Verification items for the finished model (mm, model axes). Face numbers are marked on the shaded views. A direction names the side the tool comes from. Give positions to 0.01 mm unless a question says otherwise; leave off trailing zeros. Order: outer loops, then holes, each group sorted by start corner. A loop starts at its lowest first (then second) coordinate and runs counter-clockwise, first axis right, second up. Notation, with made-up numbers: (40, 32.5) -> (74, 32.5) arc R28 cw to (74, 61.5) -> close; hole circle Ø2 at (51.5, 20). An arc over 180 degrees is marked (long way). Return JSON: item names as keys, results as strings. Group by question number.
(1) Depth check by flat-ended pin: pin 1 Ø0.8 at (y, z) = (15.5, 0) entering from +X; pin 2 Ø3 at (x, y) = (-15.5, 1) entering from -Z; pin 3 Ø1.8 at (x, y) = (5.5, 6) entering from -Z; pin 4 Ø1.4 at (x, z) = (-15.5, -0.5) entering from +Y. Enter the tip coordinate at first touch or a pass-through.
(2) Thickness scan on line 1 along Y through (x, z) = (0, -0.9); line 2 along Y through (x, z) = (0, 0.7); line 3 along X through (y, z) = (-1.25, -0.45). Record the ranges inside material, lowest first.
(3) Cross-section at B-B on x = -15.8. Enter the section's corners in (y, z).
(4) Cross-section at A-A on x = 0. Enter the section's corners in (y, z).
(5) Cross-section at D-D on z = 0.55. Enter the section's corners in (x, y), then the cut area to 3 significant figures.
(6) Release check for a two-part mould opening along X. For the marked faces 5, 6 and 7 record: pulls with the +X half, pulls with the -X half, needs draft (parallel to the pull), parting line crosses it, or undercut.
(7) Tool access check on the marked faces 1, 2, 3 and 4. Record the directions out of +Z, -Z, +X, -X, +Y, -Y that give a thin tool (end or side, any length) a straight path to the whole face; none if there is none.
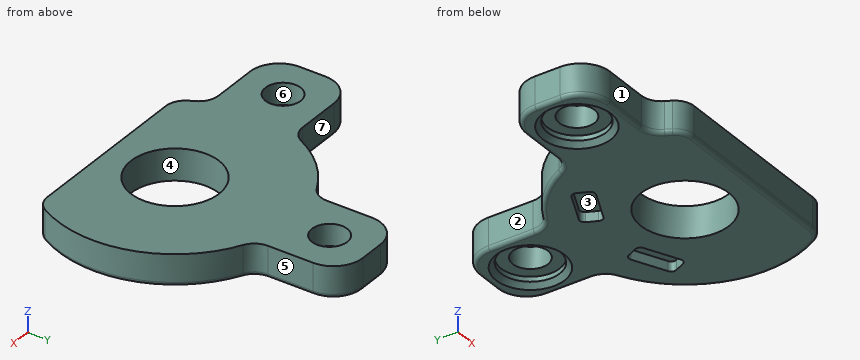
from build123d import *

# Parameters (mm, degrees)
SKETCH10_R          = 4.5
BOSS_EXTRUDE6_DEPTH = 1.6
SKETCH13_R          = 1.8
BOSS_EXTRUDE7_DEPTH = 1.6
FILLET1_R           = 2
CUT_EXTRUDE2_DEPTH  = 1
SKETCH16_R          = 3
CUT_EXTRUDE3_DEPTH  = 1
CHAMFER1_SIZE       = 0.5
FILLET2_R           = 0.4


with BuildPart() as part:
    # Sketch10 → Boss-Extrude6 (new body, symmetric)
    with BuildSketch(Plane.XY):
        with BuildLine():
            Line((-9.746794345, -7), (9.746794345, -7))
            ThreePointArc((9.746794345, -7), (0, 12), (-9.746794345, -7))
        make_face()
        Circle(SKETCH10_R, mode=Mode.SUBTRACT)
    extrude(amount=BOSS_EXTRUDE6_DEPTH, both=True)

    # Sketch13 → Boss-Extrude7 (add, symmetric)
    with BuildSketch(Plane.XY):
        with BuildLine():
            Line((-11.203124564, 4.3), (-17.1, 4.3))
            ThreePointArc((-17.1, 4.3), (-19.221320344, 3.421320344), (-20.1, 1.3))
            Line((-20.1, 1.3), (-20.1, -1.3))
            ThreePointArc((-20.1, -1.3), (-19.221320344, -3.421320344), (-17.1, -4.3))
            Line((-17.1, -4.3), (-11.203124564, -4.3))
            ThreePointArc((-11.203124564, -4.3), (-12, 0), (-11.203124564, 4.3))
        make_face()
        with Locations((-15.8, 0)):
            Circle(SKETCH13_R, mode=Mode.SUBTRACT)
        with BuildLine():
            Line((4.3, 11.203124564), (4.3, 17.1))
            ThreePointArc((4.3, 17.1), (3.421320344, 19.221320344), (1.3, 20.1))
            Line((1.3, 20.1), (-1.3, 20.1))
            ThreePointArc((-1.3, 20.1), (-3.421320344, 19.221320344), (-4.3, 17.1))
            Line((-4.3, 17.1), (-4.3, 11.203124564))
            ThreePointArc((-4.3, 11.203124564), (0, 12), (4.3, 11.203124564))
        make_face()
        with Locations((0, 15.8)):
            Circle(SKETCH13_R, mode=Mode.SUBTRACT)
    extrude(amount=BOSS_EXTRUDE7_DEPTH, both=True)

    # Fillet1
    fillet1_edges = [part.edges().sort_by_distance(p)[0] for p in [
        (-11.203124564, -4.3, 0),
        (-11.203124564, 4.3, 0),
        (-4.3, 11.203124564, 0),
        (4.3, 11.203124564, 0),
        (9.746794345, -7, 0),
        (-9.746794345, -7, 0),
    ]]
    fillet(fillet1_edges, radius=FILLET1_R)

    # Sketch15 → Cut-Extrude2 (cut)
    with BuildSketch(Plane(origin=(0, 0, -1.6), x_dir=(-1, 0, 0), z_dir=(0, 0, -1))):
        with BuildLine():
            Line((-3.808047036, 8.187368684), (-7.070755069, 6.665942941))
            ThreePointArc((-7.070755069, 6.665942941), (-7.329292249, 6.38379912), (-7.312599832, 6.001479917))
            Line((-7.312599832, 6.001479917), (-6.847719744, 5.004541351))
            ThreePointArc((-6.847719744, 5.004541351), (-6.565575922, 4.746004172), (-6.18325672, 4.762696589))
            Line((-6.18325672, 4.762696589), (-2.920548686, 6.284122331))
            ThreePointArc((-2.920548686, 6.284122331), (-2.662011507, 6.566266153), (-2.678703924, 6.948585355))
            Line((-2.678703924, 6.948585355), (-3.143584012, 7.945523921))
            ThreePointArc((-3.143584012, 7.945523921), (-3.425727833, 8.204061101), (-3.808047036, 8.187368684))
        make_face()
        with BuildLine():
            Line((6.847719744, 5.004541351), (7.312599832, 6.001479917))
            ThreePointArc((7.312599832, 6.001479917), (7.329292249, 6.38379912), (7.070755069, 6.665942941))
            Line((7.070755069, 6.665942941), (3.808047036, 8.187368684))
            ThreePointArc((3.808047036, 8.187368684), (3.425727833, 8.204061101), (3.143584012, 7.945523921))
            Line((3.143584012, 7.945523921), (2.678703924, 6.948585355))
            ThreePointArc((2.678703924, 6.948585355), (2.662011507, 6.566266153), (2.920548686, 6.284122331))
            Line((2.920548686, 6.284122331), (6.18325672, 4.762696589))
            ThreePointArc((6.18325672, 4.762696589), (6.565575922, 4.746004172), (6.847719744, 5.004541351))
        make_face()
    extrude(amount=-CUT_EXTRUDE2_DEPTH, mode=Mode.SUBTRACT)

    # Sketch16 → Cut-Extrude3 (cut)
    with BuildSketch(Plane(origin=(0, 0, -1.6), x_dir=(-1, 0, 0), z_dir=(0, 0, -1))):
        with Locations((0, 15.8)):
            Circle(SKETCH16_R)
        with Locations((15.8, 0)):
            Circle(SKETCH16_R)
    extrude(amount=-CUT_EXTRUDE3_DEPTH, mode=Mode.SUBTRACT)

    # Chamfer1
    chamfer1_edges = [part.edges().sort_by_distance(p)[0] for p in [
        (3, 15.8, -1.6),
        (-12.8, 0, -1.6),
    ]]
    chamfer(chamfer1_edges, length=CHAMFER1_SIZE)

    # Fillet2
    fillet2_edges = [part.edges().sort_by_distance(p)[0] for p in [
        (-19.221320344, 3.421320344, -1.6),
        (-20.1, 0, -1.6),
        (-19.221320344, -3.421320344, -1.6),
        (-14.801199885, -4.3, -1.6),
        (3.421320344, 19.221320344, -1.6),
        (0, 20.1, -1.6),
        (-3.421320344, 19.221320344, -1.6),
        (-4.3, 14.801199885, -1.6),
        (-14.801199885, 4.3, -1.6),
        (-8.485281374, 8.485281374, -1.6),
        (4.3, 14.801199885, -1.6),
        (11.498184685, 3.433911609, -1.6),
        (-10.558586547, -5.702302178, -1.6),
        (0, -7, -1.6),
        (-9.660254038, -6.732050808, -1.6),
        (9.660254038, -6.732050808, -1.6),
        (-11.453590921, 4.597061363, -1.6),
        (4.597061363, 11.453590921, -1.6),
        (-4.597061363, 11.453590921, -1.6),
        (-11.453590921, -4.597061363, -1.6),
    ]]
    fillet(fillet2_edges, radius=FILLET2_R)


solid = part.part
Verdict:
{
 "1": {"pin 1": "x = 4.3", "pin 2": "z = -0.6", "pin 3": "z = -1.6", "pin 4": "y = 4.3"},
 "2": {"line 1": "-7 to -4.5, 4.5 to 12.8, 18.8 to 20.1", "line 2": "-7 to -4.5, 4.5 to 14, 17.6 to 20.1", "line 3": "-20.1 to -17.1, -14.5 to -4.32, 4.32 to 11.93"},
 "3": {"outline": "(-4.3, -1.2) arc R0.4 ccw to (-3.9, -1.6) -> (-3.5, -1.6) -> (-3, -1.1) -> (-3, -0.6) -> (-1.8, -0.6) -> (-1.8, 1.6) -> (-4.3, 1.6) -> close; (1.8, -0.6) -> (3, -0.6) -> (3, -1.1) -> (3.5, -1.6) -> (3.9, -1.6) arc R0.4 ccw to (4.3, -1.2) -> (4.3, 1.6) -> (1.8, 1.6) -> close"},
 "4": {"outline": "(-7, -1.2) arc R0.4 ccw to (-6.6, -1.6) -> (-4.5, -1.6) -> (-4.5, 1.6) -> (-7, 1.6) -> close; (4.5, -1.6) -> (12.3, -1.6) -> (12.8, -1.1) -> (12.8, -0.6) -> (14, -0.6) -> (14, 1.6) -> (4.5, 1.6) -> close; (17.6, -0.6) -> (18.8, -0.6) -> (18.8, -1.1) -> (19.3, -1.6) -> (19.7, -1.6) arc R0.4 ccw to (20.1, -1.2) -> (20.1, 1.6) -> (17.6, 1.6) -> close"},
 "5": {"outline": "(-20.1, -1.3) arc R3 ccw to (-17.1, -4.3) -> (-12.5, -4.3) arc R2 cw to (-10.72, -5.4) arc R12 ccw to (-10.39, -6) arc R2 ccw to (-8.66, -7) -> (8.66, -7) arc R2 ccw to (10.39, -6) arc R12 ccw to (5.4, 10.72) arc R2 cw to (4.3, 12.5) -> (4.3, 17.1) arc R3 ccw to (1.3, 20.1) -> (-1.3, 20.1) arc R3 ccw to (-4.3, 17.1) -> (-4.3, 12.5) arc R2 cw to (-5.4, 10.72) arc R12 ccw to (-10.72, 5.4) arc R2 cw to (-12.5, 4.3) -> (-17.1, 4.3) arc R3 ccw to (-20.1, 1.3) -> close; hole circle Ø3.6 at (-15.8, 0); hole circle Ø9 at (0, 0); hole circle Ø3.6 at (0, 15.8)", "area": "437 mm²"},
 "6": {"face 5": "pulls with the +X half", "face 6": "undercut", "face 7": "needs draft"},
 "7": {"face 1": "+Z, -Z, -X, -Y", "face 2": "+Z, -Z, -X, +Y", "face 3": "-Z", "face 4": "+Z, -Z"}
}
